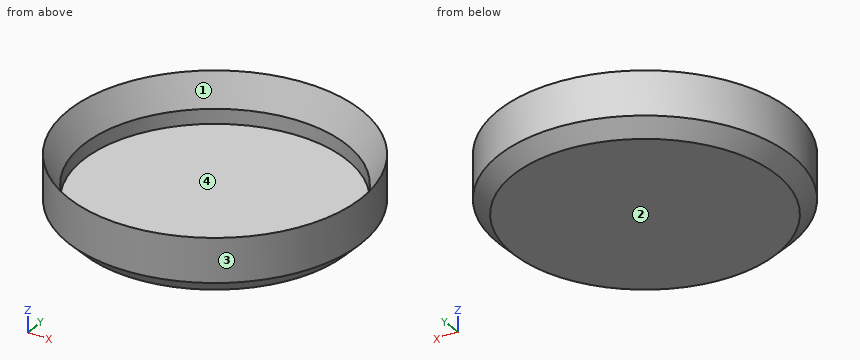
from build123d import *

# Parameters (mm, degrees)
F0_R     = 45
F1_DEPTH = 5
F0_R_2   = 50
F2_DEPTH = 20
F3_SIZE2 = 5
F3_SIZE  = 5
F4_SIZE2 = 4.99999
F4_SIZE  = 9.99999


# Not quite as in the source:
# - a fillet or chamfer is up to 0.001 mm smaller than in the source, because OpenCascade refuses the exact size
# - a feature of the source that left no trace in its solid (it failed there, or was rolled back) is left out


with BuildPart() as f1:
    # F0 (on Top) → F1 (new body)
    with BuildSketch(Plane.XY):
        Circle(F0_R)
    extrude(amount=F1_DEPTH)

    # F0 (on Top) → F2 (join)
    with BuildSketch(Plane.XY):
        Circle(F0_R_2)
        Circle(F0_R, mode=Mode.SUBTRACT)
    extrude(amount=F2_DEPTH)

    # F3
    f3_edges = [f1.edges().sort_by_distance(p)[0] for p in [
        (-50, 0, 0),
    ]]
    chamfer(f3_edges, length=F3_SIZE, length2=F3_SIZE2)

    # F4 (size 10 and 5 in the source; OpenCascade refuses exactly that, so slightly less here)
    f4_edges = [f1.edges().sort_by_distance(p)[0] for p in [
        (-45, 0, 20),
    ]]
    f4_side = f1.faces().sort_by_distance((-45, 0, 12.5))[0]
    chamfer(f4_edges, length=F4_SIZE, length2=F4_SIZE2, reference=f4_side)


solid = f1.part
Geometry check sheet. Reference: the model listing, model coordinates, mm. Face numbers are marked on the shaded views. Round coordinates to 2 decimals unless told otherwise and drop trailing zeros. Order: outer loops, then holes, each group sorted by start corner. A loop starts at its lowest first (then second) coordinate and runs counter-clockwise, first axis right, second up. Notation, with made-up numbers: M -5.75,-17.75 L 11.25,-17.75 A17 ccw 11.25,12.25 Z; hole C -25.5,18 d3. An arc over 180 degrees is marked long. Answer in a Markdown table with one row per item.
(1) Sectioned sample at C-C, the plane z = 2. Record the cut outline in (x, y).
Responses:
| item | result |
|---|---|
| outline | C 0,0 d94 |
(2) Sectioned sample at B-B, the plane z = 18. Record the cut outline in (x, y).
Responses:
| item | result |
|---|---|
| outline | C 0,0 d100; hole C 0,0 d98 |
(3) Draft check along X on the marked faces 1, 2, 3 and 4. Enter one of: released by +X, released by -X, zero draft, split by the parting line, or undercut.
Responses:
| item | result |
|---|---|
| face 1 | undercut |
| face 2 | zero draft |
| face 3 | split by the parting line |
| face 4 | undercut |
(4) Go/stop test with flat-tipped pins: P1, Ø1.5, axis at y = -37.5, z = 4, coming from the -X side; P2, Ø1, axis at x = -35.5, z = 12.5, coming from the -Y side; P3, Ø10, axis at y = -19.5, z = 2.5, coming from the +X side. Record where each tip stops, or that it passes through.
Responses:
| item | result |
|---|---|
| P1 | stops at x = -32.98 |
| P2 | stops at y = -35.71 |
| P3 | stops at x = 47.64 |
(5) Scan lines: probe 1 along Y at (x, z) = (0, 8.8); probe 2 along Z at (x, y) = (-31.5, 30); probe 3 along Y at (x, z) = (16, 7.75). Record each from-to range of solid material in increasing order. Write a range as from..to.
Responses:
| item | result |
|---|---|
| probe 1 | y = -50..-45, 45..50 |
| probe 2 | z = 0..5 |
| probe 3 | y = -47.37..-42.06, 42.06..47.37 |
